```python
from build123d import *

# Parameters (mm, degrees)
SKETCH1_R           = 50
SKETCH1_R_2         = 5
BOSS_EXTRUDE1_DEPTH = 10
SKETCH2_R           = 3.5
BOSS_EXTRUDE2_DEPTH = 25


with BuildPart() as part:
    # Sketch1 → Boss-Extrude1 (new body)
    with BuildSketch(Plane.XY):
        Circle(SKETCH1_R)
        Circle(SKETCH1_R_2, mode=Mode.SUBTRACT)
    extrude(amount=BOSS_EXTRUDE1_DEPTH)

    # Sketch2 → Boss-Extrude2 (add)
    with BuildSketch(Plane.XY.offset(10)):
        with Locations((0, 41)):
            Circle(SKETCH2_R)
        with Locations((28.991378029, 28.991378029)):
            Circle(SKETCH2_R)
        with Locations((41, 0)):
            Circle(SKETCH2_R)
        with Locations((28.991378029, -28.991378029)):
            Circle(SKETCH2_R)
        with Locations((0, -41)):
            Circle(SKETCH2_R)
        with Locations((-28.991378029, -28.991378029)):
            Circle(SKETCH2_R)
        with Locations((-41, 0)):
            Circle(SKETCH2_R)
        with Locations((-28.991378029, 28.991378029)):
            Circle(SKETCH2_R)
    extrude(amount=BOSS_EXTRUDE2_DEPTH)


solid = part.part
```
For this review, take the finished solid that the model builds, in its own axes (mm). A direction names the side the tool comes from. Coordinates: 2 decimals unless noted, no trailing zeros. Write each loop counter-clockwise with the first axis right and the second up, starting at its lowest first coordinate (ties: lowest second). Pieces come first, ordered by that corner, then holes.
(1) Wall thickness on probe 1 along Y at (x, z) = (0, 2.75); probe 2 along Z at (x, y) = (9.5, -1); probe 3 along Y at (x, z) = (32, 24): over which ranges is each line inside the solid? List them lowest first.
(2) The part is to be moulded in two halves that separate along Y. For faces 3 (the face through (-44.497, 0.154, 22.325)), 4 (the face through (41, 0, 35)), 5 (the face through (26.412, 31.357, 22.325)), say which applies: +Y half, -Y half, draft (parallel to the pull), parting line (faces both ways), or undercut.
(3) Tool access review of faces 1 (the face through (0, 41, 35)), 2 (the face through (-1, -10, 10)): name each direction out of +Z, -Z, +X, -X, +Y, -Y from which nothing blocks a thin tool from reaching the whole face with its end or side.
(4) For pin 1 Ø9 at (x, y) = (0, 0) entering from -Z; pin 2 Ø5 at (y, z) = (-31.5, 22.5) entering from +X; pin 3 Ø12 at (x, z) = (-10.5, 12.5) entering from +Y; pin 4 Ø8 at (y, z) = (-31.5, 12) entering from -X, all flat-tipped, find the tip position at first contact; note any pin that passes through.
(5) Add section D-D on x = 29. Give the boundary of the cut face in (y, z).
(6) Add section A-A on y = 0. Give the boundary of the cut face in (x, z).
(7) Add section C-C on z = 26. Give the boundary of the cut face in (x, y), then the cut area to 3 significant figures.
Answer sheet:
1. probe 1: y = -50 to -5, 5 to 50
1. probe 2: z = 0 to 10
1. probe 3: y = -30.78 to -27.2, 27.2 to 30.78
2. face 3: parting line
2. face 4: draft
2. face 5: undercut
3. face 1: +Z, +X, -X, +Y, -Y
3. face 2: +Z
4. pin 1: passes through
4. pin 2: stops at x = 32.49
4. pin 3: stops at y = 49.74
4. pin 4: stops at x = -41.4
5. outline: (-40.73, 0) - (40.73, 0) - (40.73, 10) - (32.49, 10) - (32.49, 35) - (25.49, 35) - (25.49, 10) - (-25.49, 10) - (-25.49, 35) - (-32.49, 35) - (-32.49, 10) - (-40.73, 10) - close
6. outline: (-50, 0) - (-5, 0) - (-5, 10) - (-37.5, 10) - (-37.5, 35) - (-44.5, 35) - (-44.5, 10) - (-50, 10) - close; (5, 0) - (50, 0) - (50, 10) - (44.5, 10) - (44.5, 35) - (37.5, 35) - (37.5, 10) - (5, 10) - close
7. outline: circle Ø7 at (-41, 0); circle Ø7 at (-28.99, -28.99); circle Ø7 at (-28.99, 28.99); circle Ø7 at (0, -41); circle Ø7 at (0, 41); circle Ø7 at (28.99, -28.99); circle Ø7 at (28.99, 28.99); circle Ø7 at (41, 0)
7. area: 308 mm2
